```python
from build123d import *

# Parameters (mm, degrees)
SKETCH1_R           = 45
BOSS_EXTRUDE1_DEPTH = 50


with BuildPart() as part:
    # Sketch1 → Boss-Extrude1 (new body)
    with BuildSketch(Plane(origin=(0, 0, 0), x_dir=(1, 0, 0), z_dir=(0, 1, 0))):
        Circle(SKETCH1_R)
    extrude(amount=BOSS_EXTRUDE1_DEPTH)

    # Sketch2 → Cut-Revolve1 (revolve, cut)
    with BuildSketch(Plane(origin=(0, 0, 0), x_dir=(0, 0, -1), z_dir=(1, 0, 0))):
        Polygon((0, 50), (0, 0), (-40, 0), (-40, 10), (-37, 10), (-6, 41), (-6, 50), align=None)
    revolve(axis=Axis((0, 50, 0), (0, -1, 0)), mode=Mode.SUBTRACT)

    # Sketch3 → Revolve1 (revolve)
    with BuildSketch(Plane(origin=(0, 0, 0), x_dir=(0, 0, -1), z_dir=(1, 0, 0))):
        Polygon((-6, 50), (-20.522939955, 50), (-20.522939955, 70), (-6, 70), (-2.249869877, 61), (-2.249869877, 59), align=None)
    revolve(axis=Axis((0, 70, 0), (0, -1, 0)))


solid = part.part
```
Design review of the part built by this model. Coordinates are the model's own, in mm. A direction names the side the tool comes from. Coordinates: 2 decimals unless noted, no trailing zeros. Order: outer loops, then holes, each group sorted by start corner. A loop starts at its lowest first (then second) coordinate and runs counter-clockwise, first axis right, second up. Notation, with made-up numbers: (16.25, -29) -> (74.25, -29) arc R18 ccw to (74.25, -16) -> close; hole circle Ø4 at (52, 69.5). An arc over 180 degrees is marked (long way). One line per item, written item: value. Start each with the question number.
Q1. Take a section at C-C, the plane y = 24.5. State the section outline as (x, z) points, then the cut area to 3 significant figures.
Q2. Insertion check: pin 1 Ø10 at (x, z) = (21, 15.5) entering from -Y; pin 2 Ø15.5 at (x, z) = (0, 0) entering from +Y; pin 3 Ø8 at (y, z) = (9, -25) entering from -X; pin 4 Ø5 at (x, z) = (0, 0) entering from -Y. Each pin has a flat end and moves straight along its axis. Give the tip position at first contact, or say it passes through.
Q3. Tool access review of faces 1 (the flat face through (35.4, 10, 11.7)), 2 (the flat face through (-30.2, 0, 26.5)), 3 (the flat face through (9, 50, 19)): name each direction out of +Z, -Z, +X, -X, +Y, -Y from which nothing blocks a thin tool from reaching the whole face with its end or side.
Q4. For probe 1 along X at (y, z) = (60, 0); probe 2 along Z at (x, y) = (0, 45.75); probe 3 along Z at (x, y) = (0, 6.5), list the stretches that pass through material, from the lowest coordinate up.
Q5. Take a section at D-D, the plane y = 16. State the section outline as (x, z) points, then the cut area to 3 significant figures.
Q6. Take a section at A-A, the plane x = 0. State the section outline as (y, z) points, then the cut area to 3 significant figures.
Q7. Mouldability with a two-part tool opening along Z and no side actions: class faces 4 (the cylindrical face through (18.207, 60.14, 9.47)), 5 (the flat face through (-5, 70, 4)), 6 (the conical face through (2.24, 64.437, -2.922)) as pulls with the +Z half, pulls with the -Z half, needs draft (parallel to the pull), parting line crosses it, or undercut.
Q8. Take a section at B-B, the plane z = 0. State the section outline as (x, y) points, then the cut area to 3 significant figures.
Values follow:
1. outline: circle Ø90 at (0, 0); hole circle Ø45 at (0, 0)
1. area: 4,770 mm2
2. pin 1: stops at y = 15.9
2. pin 2: stops at y = 70
2. pin 3: stops at x = -39.8
2. pin 4: stops at y = 58.4
3. face 1: -Y
3. face 2: +Z, -Z, +X, -X, -Y
3. face 3: +Y
4. probe 1: x = -20.52 to -2.25, 2.25 to 20.52
4. probe 2: z = -45 to -6, 6 to 45
4. probe 3: z = -45 to -40, 40 to 45
5. outline: circle Ø90 at (0, 0); hole circle Ø62 at (0, 0)
5. area: 3,340 mm2
6. outline: (0, -45) -> (50, -45) -> (50, -20.52) -> (70, -20.52) -> (70, -6) -> (61, -2.25) -> (59, -2.25) -> (50, -6) -> (41, -6) -> (10, -37) -> (10, -40) -> (0, -40) -> close; (0, 40) -> (10, 40) -> (10, 37) -> (41, 6) -> (50, 6) -> (59, 2.25) -> (61, 2.25) -> (70, 6) -> (70, 20.52) -> (50, 20.52) -> (50, 45) -> (0, 45) -> close
6. area: 2,920 mm2
7. face 4: parting line crosses it
7. face 5: needs draft
7. face 6: undercut
8. outline: (-45, 0) -> (-40, 0) -> (-40, 10) -> (-37, 10) -> (-6, 41) -> (-6, 50) -> (-2.25, 59) -> (-2.25, 61) -> (-6, 70) -> (-20.52, 70) -> (-20.52, 50) -> (-45, 50) -> close; (2.25, 59) -> (6, 50) -> (6, 41) -> (37, 10) -> (40, 10) -> (40, 0) -> (45, 0) -> (45, 50) -> (20.52, 50) -> (20.52, 70) -> (6, 70) -> (2.25, 61) -> close
8. area: 2,920 mm2
